Input: dimensioned drawing with shaded views. Units: mm. Origin: part minimum x, y, z. A direction names the side the tool comes from. Round coordinates to 2 decimals unless told otherwise and drop trailing zeros. Order: outer loops, then holes, each group sorted by start corner. A loop starts at its lowest first (then second) coordinate and runs counter-clockwise, first axis right, second up. Notation, with made-up numbers: M 36,46 L 55,46 A8 ccw 55,53 Z; hole C 15.25,86.5 d4. An arc over 180 degrees is marked long. Use one line per item in the form item = value. Start each with the question number.
Q1. Section C-C (x = 154). Return the cut outline in (y, z).
Q2. Section D-D (z = 145). Return the cut outline in (x, y), plus the area to 3 significant figures.
Q3. Section B-B (z = 30). Return the cut outline in (x, y).
Q4. Material intervals for probe 1 along Y at (x, z) = (48, 12); probe 2 along X at (y, z) = (40, 18); probe 3 along Z at (x, y) = (222.5, 163), sorted ascending.
Q5. Reachability of the marked faces 1, 2, 3, 4 and 5 from +Z, -Z, +X, -X, +Y, -Y: full face, straight path, thin tool, end or side. Return the list, or none.
Q6. Section A-A (y = 160). Return the cut outline in (x, z).
Q7. Contact query for flat-ended pins moving along their axis: pin 1 (24 mm diameter, centred on y = 140.5, z = 117, fed in from -X); pin 2 (5 mm diameter, centred on x = 219, z = 133, fed in from +Y); pin 3 (10 mm diameter, centred on y = 106, z = 181.5, fed in from -X) (3 decimals). Output: stop coordinate, or through.
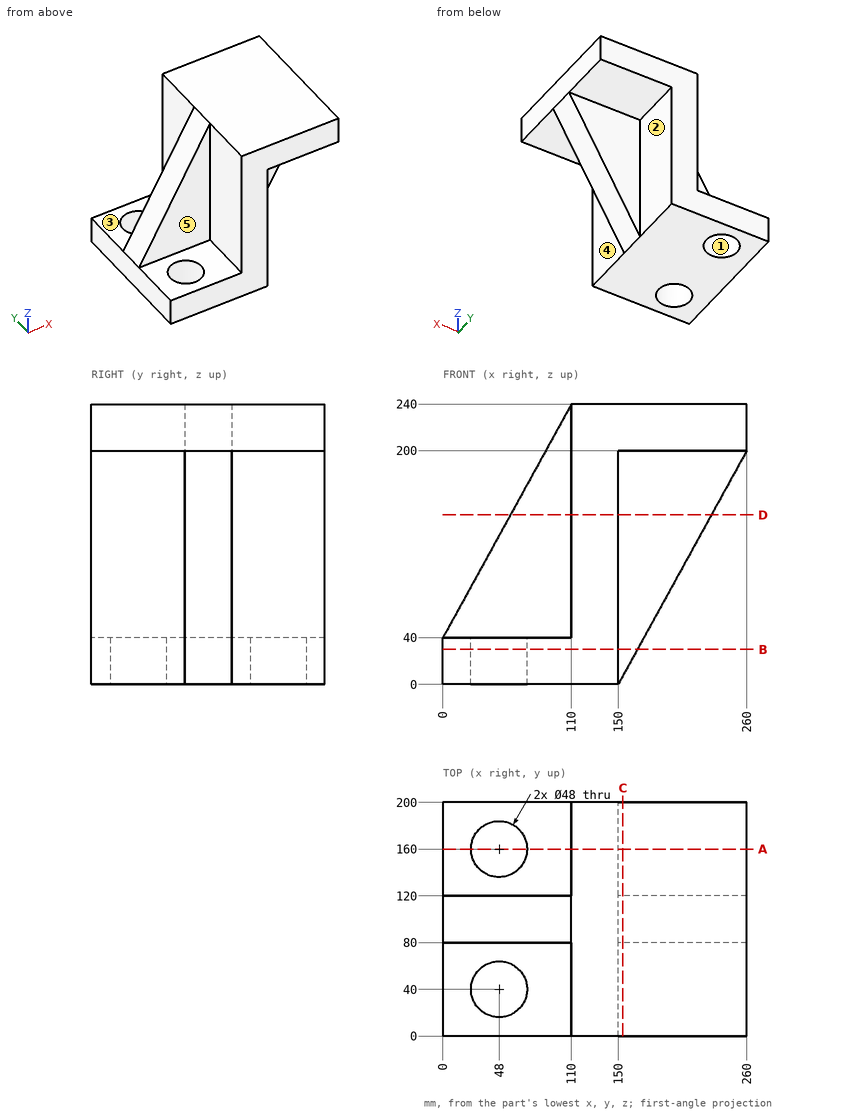
Results list:
q1.outline = M 0,200 L 80,200 L 80,7.27 L 120,7.27 L 120,200 L 200,200 L 200,240 L 0,240 Z
q2.outline = M 57.75,80 L 110,80 L 110,0 L 150,0 L 150,80 L 229.75,80 L 229.75,120 L 150,120 L 150,200 L 110,200 L 110,120 L 57.75,120 Z
q2.area = 13,300 mm2
q3.outline = M 0,0 L 150,0 L 150,80 L 166.5,80 L 166.5,120 L 150,120 L 150,200 L 0,200 Z; hole C 48,40 d48; hole C 48,160 d48
q4.probe_1 = 0 to 16, 64 to 136, 184 to 200
q4.probe_2 = 0 to 24, 72 to 150
q4.probe_3 = 200 to 240
q5.face_1 = +Z, -Z
q5.face_2 = -Z, +X, +Y
q5.face_3 = +Z, -X, +Y
q5.face_4 = -Z, +X, -Y
q5.face_5 = +Z, -X, -Y
q6.outline = M 0,0 L 24,0 L 24,40 L 0,40 Z; M 72,0 L 150,0 L 150,200 L 260,200 L 260,240 L 110,240 L 110,40 L 72,40 Z
q7.pin_1 = 110
q7.pin_2 = 120
q7.pin_3 = 75.075
